Check sheet for the modelled part. Datum: model origin and axes. Units: mm. Face numbers are marked on the shaded views. A direction names the side the tool comes from. Coordinates: 2 decimals unless noted, no trailing zeros. Write each loop counter-clockwise with the first axis right and the second up, starting at its lowest first coordinate (ties: lowest second). Pieces come first, ordered by that corner, then holes. Notation, with made-up numbers: M -9,59 L 6,59 A26 cw 6,98 Z; hole C -37,66.5 d11. An arc over 180 degrees is marked long. Answer as CSV lines item,"result".
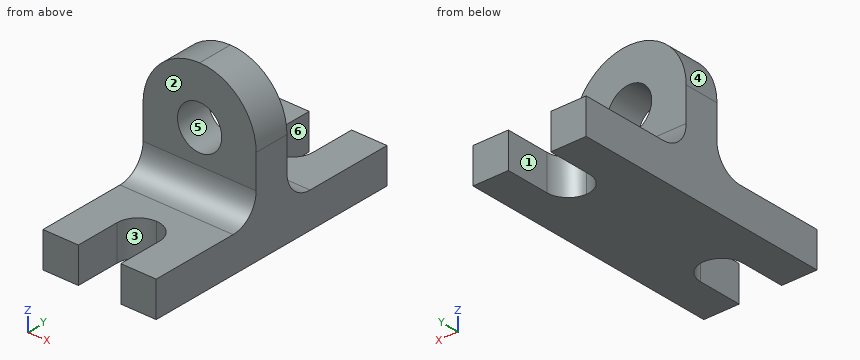
Autodesk Fusion 360 part; units mm, degrees
sketch "Sketch1" plane through (0, 0, 0) normal (0, 0, 1) x (1, 0, 0)
  line L0 (-32, 75) -> (32, 75)
  line L1 (32, 75) -> (32, -75)
  line L2 (32, -75) -> (-32, -75)
  line L3 (-32, -75) -> (-32, 75)
  line L4 (-32, -10) -> (32, -10)
  line L5 (32, -10) -> (32, 10)
  line L6 (32, 10) -> (-32, 10)
  line L7 (-32, 10) -> (-32, -10)
  line L8 (-12, 75) -> (12, 75)
  line L9 (12, 75) -> (12, 38)
  line L10 (12, 38) -> (-12, 38)
  line L11 (-12, 38) -> (-12, 75)
  line L12 (-32, 0) -> (32, 0)
  line L13 (-12, -38) -> (-12, -75)
  line L14 (12, -38) -> (-12, -38)
  line L15 (12, -75) -> (12, -38)
  dimension "d1" = 64
  dimension "d2" = 150
  dimension "d3" = 75
  dimension "d4" = 32
  dimension "d5" = 20
  dimension "d6" = 10
  dimension "d7" = 24
  dimension "d8" = 37
  dimension "d9" = 12
extrude "Extrude1" add sketch "Sketch1" along normal blind 20 contours L0 L1 L3 L6 L9 L10 L11 | L1 L2 L3 L4 L13 L14 L15 makes body 1 at (-4, -19.3333, 0) makes body 2 at (4, 19.3333, 0)
extrude "Extrude2" add sketch "Sketch1" along normal blind 86 contours L1 L3 L5 L6 L7 L12 | L1 L3 L4 L5 L7 L12 bodies 1 2
sketch "Sketch2" plane through (0, -10, 0) normal (0, -1, 0) x (1, 0, 0)
  line L0 (-32, 20) -> (32, 20)
  line L1 (32, 20) -> (32, 86)
  line L2 (32, 86) -> (-32, 86)
  line L3 (-32, 86) -> (-32, 20)
  circle A0 centre (0, 54) radius 12.5
  line L4 (32, 0) -> (-32, 0)
  dimension "d14" = 25
  dimension "d16" = 54
extrude "Extrude3" cut sketch "Sketch2" against normal up to surface (20 mm away) contours A0 bodies 1
fillet "Fillet1" radius 32 2 edges at (32, 0, 86) (-32, 0, 86) on bodies 1
fillet "Fillet2" radius 15 2 edges at (0, 10, 20) (0, -10, 20) on bodies 1
fillet "Fillet3" radius 12 4 edges at (-12, -38, 10) (12, -38, 10) (12, 38, 10) (-12, 38, 10) on bodies 1
equation "d1 = ( 2 * 20 ) * 1 mm + 24 mm"
equation "d2 = ( 2 * 65 ) * 1 mm + 20 mm"
equation "d3 = ( 150 / 2 ) * 1 mm"
equation "d8 = 25 mm + 12 mm"
equation "d12 = 54 mm + 32 mm"
1) Section check D-D, the plane z = 69.5. Record the boundary of the cut face in (x, y), plus the area to 3 significant figures.
Answer key:
outline,"M -28,-10 L 28,-10 L 28,10 L -28,10 Z"
area,"1,120 mm2"
2) Section check B-B, the plane z = 47. Record the boundary of the cut face in (x, y), plus the area to 3 significant figures.
Answer key:
outline,"M -32,-10 L -10.36,-10 L -10.36,10 L -32,10 Z; M 10.36,-10 L 32,-10 L 32,10 L 10.36,10 Z"
area,"866 mm2"
3) Thickness scan on line 1 along Z through (x, y) = (0, 0); line 2 along Y through (x, z) = (-17.5, 77); line 3 along X through (y, z) = (44.5, 10.5). Record the ranges inside material, lowest first.
Answer key:
line 1,"z = 0 to 41.5, 66.5 to 86"
line 2,"y = -10 to 10"
line 3,"x = -32 to -10.67, 10.67 to 32"
4) Mould release check, pull along Z, two halves, no side actions. Record for the marked faces 4, 5 and 6: pulls with the +Z half, pulls with the -Z half, needs draft (parallel to the pull), parting line crosses it, or undercut.
Answer key:
face 4,"pulls with the +Z half"
face 5,"undercut"
face 6,"needs draft"
5) Depth check by flat-ended pin: P1, Ø15, axis at x = -1, y = 44, coming from the +Z side; P2, Ø2, axis at x = -10, z = 64.5, coming from the -Y side; P3, Ø5, axis at x = -13, z = 28, coming from the +Y side. Enter the tip coordinate at first touch or a pass-through.
Answer key:
P1,"stops at z = 20"
P2,"stops at y = -10"
P3,"stops at y = 13.39"
6) Section check A-A, the plane y = 54.5. Record the boundary of the cut face in (x, z), plus the area to 3 significant figures.
Answer key:
outline,"M -32,0 L -12,0 L -12,20 L -32,20 Z; M 12,0 L 32,0 L 32,20 L 12,20 Z"
area,"800 mm2"
7) Tool access check on the marked faces 1, 2 and 3. Record the directions out of +Z, -Z, +X, -X, +Y, -Y that give a thin tool (end or side, any length) a straight path to the whole face; none if there is none.
Answer key:
face 1,"+Z, -Z, +Y"
face 2,"+Z, +X, -X, -Y"
face 3,"+Z, -Z, -Y"
8) Section check C-C, the plane y = -34. Record the boundary of the cut face in (x, z).
Answer key:
outline,"M -32,0 L 32,0 L 32,20 L -32,20 Z"
